```python
from build123d import *

# Parameters (mm, degrees)
SKETCH1_W           = 2.8702
SKETCH1_H           = 3.5052
SKETCH2_R           = 1.7526
BOSS_EXTRUDE1_DEPTH = 31.75
CUT_EXTRUDE1_DEPTH  = 1.6256
CHAMFER1_SIZE       = 0.47244
CHAMFER2_SIZE       = 0.3556
FILLET1_R           = 0.254


with BuildPart() as part:
    # Sketch1 → Revolve1 (revolve)
    with BuildSketch(Plane.XY):
        with Locations((1.4351, 1.7526)):
            Rectangle(SKETCH1_W, SKETCH1_H)
    revolve(axis=Axis((0, 3.5052, 0), (0, -1, 0)))

    # Sketch2 → Boss-Extrude1 (add)
    with BuildSketch(Plane.XZ):
        Circle(SKETCH2_R)
    extrude(amount=BOSS_EXTRUDE1_DEPTH)

    # Sketch3 → Cut-Extrude1 (cut)
    with BuildSketch(Plane(origin=(0, 3.5052, 0), x_dir=(-1, 0, 0), z_dir=(0, 1, 0))):
        Polygon((-0.799225978, 1.3843), (-1.598451955, 0), (-0.799225978, -1.3843), (0.799225978, -1.3843), (1.598451955, 0), (0.799225978, 1.3843), align=None)
    extrude(amount=-CUT_EXTRUDE1_DEPTH, mode=Mode.SUBTRACT)

    # Sketch4 → Cut-Revolve1 (revolve, cut)
    with BuildSketch(Plane.XY):
        Polygon((1.3843, 1.8796), (0, 1.8796), (0, 1.080374022), align=None)
    revolve(axis=Axis((0, 1.879625, 0), (0, -1, 0)), mode=Mode.SUBTRACT)

    # Chamfer1
    chamfer1_edges = [part.edges().sort_by_distance(p)[0] for p in [
        (-1.7526, -31.75, 0),
    ]]
    chamfer(chamfer1_edges, length=CHAMFER1_SIZE)

    # Chamfer2
    chamfer2_edges = [part.edges().sort_by_distance(p)[0] for p in [
        (-2.8702, 3.5052, 0),
    ]]
    chamfer(chamfer2_edges, length=CHAMFER2_SIZE)

    # Fillet1
    fillet1_edges = [part.edges().sort_by_distance(p)[0] for p in [
        (-1.7526, 0, 0),
    ]]
    fillet(fillet1_edges, radius=FILLET1_R)


solid = part.part
```
Model file for the job. Use its own axes, mm. A direction names the side the tool comes from. Round coordinates to 2 decimals unless told otherwise and drop trailing zeros. Write each loop counter-clockwise with the first axis right and the second up, starting at its lowest first coordinate (ties: lowest second). Pieces come first, ordered by that corner, then holes. Notation, with made-up numbers: M -22,-19 L -9,-19 A14 cw -9,2 Z; hole C 20.25,-17 d7. An arc over 180 degrees is marked long. Put each result on its own line as item: value.
Item 1: Probe L1, parallel to X at y = -21.5, z = -0.1; L2, parallel to X at y = 1, z = 0.2; L3, parallel to Y at x = 1.9, z = 1.6. List the from-to ranges inside material, lowest first. Write a range as from..to.
Responses:
L1: -1.75..1.75
L2: -2.86..2.86
L3: 0..3.51
Item 2: Tool access for faces 4 (the cylindrical face through (1.67, -15.55, 0.53)), 5 (the flat face through (0, -31.75, 0)), 6 (the flat face through (1.193, 2.704, 0.702)): list every direction of +Z, -Z, +X, -X, +Y, -Y with a clear straight run to the whole face (end or side of a thin tool).
Responses:
face 4: -Y
face 5: +Z, -Z, +X, -X, -Y
face 6: +Y
Item 3: Flat gauge pins, fed straight in: P1, Ø1.5, axis at x = 1.5, z = 1, coming from the -Y side; P2, Ø2, axis at y = -9.5, z = 1.5, coming from the +X side; P3, Ø2, axis at x = -0.5, y = -8.5, coming from the +Z side; P4, Ø0.6, axis at x = -0.5, z = 1, coming from the +Y side. Where does each tip first touch, or does it go through?
Responses:
P1: y = -31.75
P2: x = 1.68
P3: z = 1.75
P4: y = 1.88
Item 4: Mould opens along Z. For faces 1 (the cylindrical face through (-2.278, 1.597, -1.746)), 2 (the conical face through (0.111, 1.219, -0.213)), 3 (the flat face through (0, 3.505, -2)) say: +Z half, -Z half, draft (parallel to the pull), parting line (faces both ways), or undercut.
Responses:
face 1: parting line
face 2: undercut
face 3: draft
Item 5: Cut at A-A (y = -18). List the corners of the cut face in (x, z), and give its area (3 significant figures).
Responses:
outline: C 0,0 d3.51
area: 9.65 mm²
